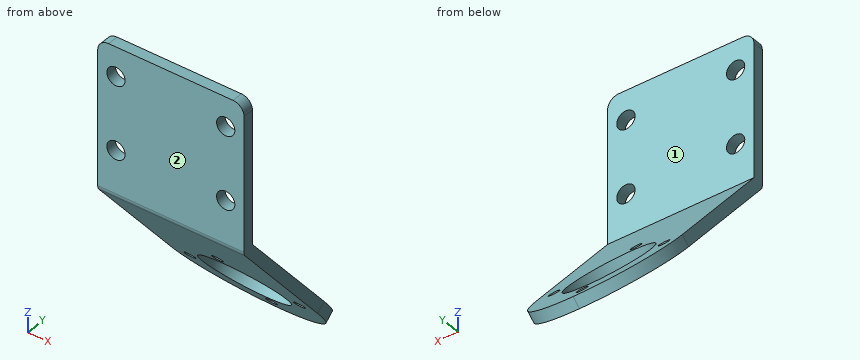
from build123d import *

# Parameters (mm, degrees)
EXTRUDE_1_DEPTH     = 40
SKETCH_3_R          = 2.5
SKETCH_3_R_2        = 2.499999999
CUT_EXTRUDE_1_DEPTH = 40
FILLET_1_R          = 3
FILLET_2_R          = 3
FILLET_3_R          = 20
FILLET_4_R          = 20
SKETCH_4_R          = 11.55
SKETCH_4_R_2        = 1.5
CUT_EXTRUDE_2_DEPTH = 40
FILLET_5_R          = 2


with BuildPart() as part:
    # 草图1 → 凸台-拉伸1 (new body)
    with BuildSketch(Plane(origin=(0, 0, 0), x_dir=(0, 0, -1), z_dir=(1, 0, 0))):
        Polygon((-39.408089297, 0), (0, 0), (45.892258904, 38.50817752), (47.820621733, 36.210044191), (1.091910703, -3), (0.178974486, -3), (-39.408089297, -3), align=None)
    extrude(amount=EXTRUDE_1_DEPTH)

    # 草图3 → 切除-拉伸1 (cut)
    with BuildSketch(Plane(origin=(0, 0, 0), x_dir=(1, 0, 0), z_dir=(0, 1, 0))):
        with Locations(Location((5, -31.408089297, 0), (0, 0, 270))):
            Circle(SKETCH_3_R)
        with Locations(Location((5, -11.408089297, 0), (0, 0, 270))):
            Circle(SKETCH_3_R_2)
        with Locations(Location((35, -11.408089297, 0), (0, 0, 270))):
            Circle(SKETCH_3_R_2)
        with Locations(Location((35, -31.408089297, 0), (0, 0, 270))):
            Circle(SKETCH_3_R)
    extrude(amount=-CUT_EXTRUDE_1_DEPTH, mode=Mode.SUBTRACT)

    # 圆角1
    fillet_1_edges = [part.edges().sort_by_distance(p)[0] for p in [
        (40, -1.5, 39.408089297),
    ]]
    fillet(fillet_1_edges, radius=FILLET_1_R)

    # 圆角2
    fillet_2_edges = [part.edges().sort_by_distance(p)[0] for p in [
        (0, -1.5, 39.408089297),
    ]]
    fillet(fillet_2_edges, radius=FILLET_2_R)

    # 圆角3
    fillet_3_edges = [part.edges().sort_by_distance(p)[0] for p in [
        (0, 37.359110856, -46.856440319),
    ]]
    fillet(fillet_3_edges, radius=FILLET_3_R)

    # 圆角4
    fillet_4_edges = [part.edges().sort_by_distance(p)[0] for p in [
        (40, 37.359110856, -46.856440319),
    ]]
    fillet(fillet_4_edges, radius=FILLET_4_R - 0.0001)  # a hair under: the kernel refuses the full size

    # 草图4 → 切除-拉伸2 (cut)
    with BuildSketch(Plane(origin=(0, 0, 0), x_dir=(1, 0, 0), z_dir=(0, 0.7660444431189773, 0.6427876096865403))):
        with Locations(Location((20, 39.908089297, 0), (0, 0, 270))):
            Circle(SKETCH_4_R)
        with Locations(Location((20, 54.908089297, 0), (0, 0, 270))):
            Circle(SKETCH_4_R_2)
        with Locations(Location((35, 39.908089297, 0), (0, 0, 270))):
            Circle(SKETCH_4_R_2)
        with Locations(Location((5, 39.908089297, 0), (0, 0, 270))):
            Circle(SKETCH_4_R_2)
        with Locations(Location((20, 24.908089297, 0), (0, 0, 270))):
            Circle(SKETCH_4_R_2)
    extrude(amount=-CUT_EXTRUDE_2_DEPTH, mode=Mode.SUBTRACT)

    # 圆角5
    fillet_5_edges = [part.edges().sort_by_distance(p)[0] for p in [
        (20, -3, -1.091910703),
    ]]
    fillet(fillet_5_edges, radius=FILLET_5_R)


solid = part.part
For this review, take the finished solid that the model builds, in its own axes (mm). Face numbers are marked on the shaded views. A direction names the side the tool comes from. Round coordinates to 2 decimals unless told otherwise and drop trailing zeros. Order: outer loops, then holes, each group sorted by start corner. A loop starts at its lowest first (then second) coordinate and runs counter-clockwise, first axis right, second up. Notation, with made-up numbers: (64.5, 82) -> (72.5, 82) arc R34 ccw to (72.5, 113) -> close; hole circle Ø1 at (17, 48). An arc over 180 degrees is marked (long way). Write item = value, one per line. Start each with the question number.
1) Take a section at A-A on x = 23. State the section outline as (y, z) points, plus the area to 3 significant figures.
2) Take a section at D-D on z = -11.5. State the section outline as (x, y) points.
3) Insertion check: pin 1 (4 mm diameter, centred on x = 11, z = 24.5, fed in from +Y); pin 2 (6 mm diameter, centred on x = 5, z = -33, fed in from -Y). Each pin has a flat end and moves straight along its axis. Give the tip position at first contact, or say it passes through.
4) Take a section at B-B on x = 5. State the section outline as (y, z) points.
5) Take a section at C-C on z = 25.5. State the section outline as (x, y) points, plus the area to 3 significant figures.
6) Tool access review of the marked faces 1 and 2: name each direction out of +Z, -Z, +X, -X, +Y, -Y from which nothing blocks a thin tool from reaching the whole face with its end or side.
7) To check wall thickness, follow line 1 (Y direction, x = 25, z = 14); line 2 (Y direction, x = 27.5, z = -7); line 3 (Z direction, x = 17.5, y = 15). State the ranges of each line that lie inside material, in increasing order. Write a range as from..to.
Verdict:
q1.outline = (-3, -0.36) arc R2 ccw to (-2.53, -1.65) -> (16.18, -23.96) -> (18.48, -22.03) -> (0, 0) -> (0, 39.41) -> (-3, 39.41) -> close; (30.52, -41.04) -> (36.06, -47.65) -> (38.36, -45.72) -> (32.82, -39.12) -> close
q1.area = 234 mm2
q2.outline = (0, 5.73) -> (40, 5.73) -> (40, 9.65) -> (0, 9.65) -> close
q3.pin_1 = 0
q3.pin_2 = 21.26
q4.outline = (-3, -0.36) arc R2 ccw to (-2.53, -1.65) -> (22.39, -31.35) -> (24.69, -29.42) -> (0, 0) -> (0, 8.91) -> (-3, 8.91) -> close; (-3, 13.91) -> (0, 13.91) -> (0, 28.91) -> (-3, 28.91) -> close; (-3, 33.91) -> (0, 33.91) -> (0, 39.41) -> (-3, 39.41) -> close; (24.32, -33.65) -> (31.86, -42.63) -> (34.16, -40.71) -> (26.62, -31.72) -> close
q5.outline = (0, -3) -> (40, -3) -> (40, 0) -> (0, 0) -> close
q5.area = 120 mm2
q6.face_1 = +Z, +X, -X, +Y
q6.face_2 = +Z, -Z, +X, -X, -Y
q7.line_1 = -3..0
q7.line_2 = 1.96..5.87
q7.line_3 = -22.54..-17.88
